from build123d import *

# Parameters (mm, degrees)
SKETCH1_R               = 2.54
BOSS_EXTRUDE1_DEPTH     = 3.175
CUT_EXTRUDE1_DEPTH      = 114.310823319
CUT_EXTRUDE1_DEPTH_BACK = 114.310823319


with BuildPart() as part:
    # Sketch1 → Boss-Extrude1 (new body)
    with BuildSketch(Plane(origin=(0, 0, 0), x_dir=(1, 0, 0), z_dir=(0, 1, 0))):
        with BuildLine():
            Line((108.539117009, 4.335152614), (5.263477484, 12.318590912))
            ThreePointArc((5.263477484, 12.318590912), (3.157372026, 12.484449553), (1.051753091, 12.656374498))
            ThreePointArc((1.051753091, 12.656374498), (-12.7, 0), (1.051753091, -12.656374498))
            ThreePointArc((1.051753091, -12.656374498), (3.157372026, -12.484449553), (5.263477484, -12.318590912))
            Line((5.263477484, -12.318590912), (108.539117009, -4.335152614))
            ThreePointArc((108.539117009, -4.335152614), (112.55208597, 0), (108.539117009, 4.335152614))
        make_face()
        with Locations(Location((108.204, 0, 0), (0, 0, 270))):
            Circle(SKETCH1_R, mode=Mode.SUBTRACT)
        with Locations(Location((96.52, 0, 0), (0, 0, 270))):
            Circle(SKETCH1_R, mode=Mode.SUBTRACT)
        with Locations(Location((84.836, 0, 0), (0, 0, 270))):
            Circle(SKETCH1_R, mode=Mode.SUBTRACT)
    extrude(amount=BOSS_EXTRUDE1_DEPTH)

    # Sketch3 → Cut-Extrude1 (cut, two sides: drawn at the far end of the back side and taken through both)
    with BuildSketch(Plane(origin=(0, 0, 0), x_dir=(1, 0, 0), z_dir=(0, 1, 0)).offset(-CUT_EXTRUDE1_DEPTH_BACK)):
        with BuildLine():
            Line((-4.018100173, 8.636), (4.018100173, 8.636))
            ThreePointArc((4.018100173, 8.636), (0, -9.525), (-4.018100173, 8.636))
        make_face()
    extrude(amount=CUT_EXTRUDE1_DEPTH + CUT_EXTRUDE1_DEPTH_BACK, mode=Mode.SUBTRACT)


solid = part.part
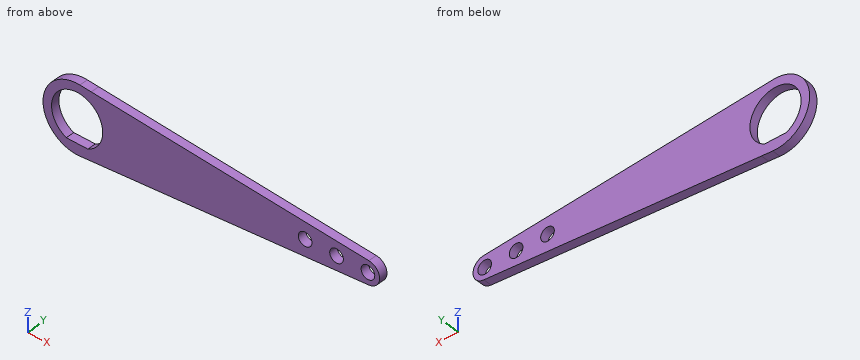
The model under review builds one solid part; all positions refer to its coordinate system, in mm. Give positions to 0.01 mm unless a question says otherwise; leave off trailing zeros. Loops run counter-clockwise (first coordinate to the right, second up) from the corner with the lowest first, then second, coordinate; pieces in that order, holes last. Notation, with made-up numbers: (-33.75, 2.5) -> (3.25, 2.5) arc R15 ccw to (3.25, 25.5) -> close; hole circle Ø9 at (15.5, -20). An arc over 180 degrees is marked (long way). Answer as a JSON object with one key per item and string values. Group by question number.
Q1. Take a section at D-D (z = 6.75). Write out the cut boundary in (x, y) (3 decimals), plus the area to 3 significant figures.
Q2. Wall thickness on line 1 along X through (y, z) = (1.2, 0) (3 decimals); line 2 along X through (y, z) = (2.2, 2); line 3 along Z through (x, y) = (0, 0.9) (3 decimals): over which ranges is each line inside the solid? List them lowest first.
Q3. Insertion check: pin 1 (8 mm diameter, centred on x = 96.52, z = 0, fed in from -Y); pin 2 (1.5 mm diameter, centred on y = 1.5, z = 1.5, fed in from +X); pin 3 (1.6 mm diameter, centred on x = -1.5, y = 2.5, fed in from +Z); pin 4 (1.5 mm diameter, centred on x = 50.5, y = 1.5, fed in from -Z). Each pin has a flat end and moves straight along its axis. Give the tip position at first contact, or say it passes through.
Q4. Take a section at A-A (x = 0). Write out the cut boundary in (y, z) (3 decimals).
Q5. Take a section at B-B (z = 0). Write out the cut boundary in (x, y) (3 decimals).
Q6. Take a section at C-C (y = 2.65). Write out the cut boundary in (x, z) (3 decimals), plus the area to 3 significant figures.
Answer below:
{
 "1": {"outline": "(-10.758, 0) -> (-6.72, 0) -> (-6.72, 3.175) -> (-10.758, 3.175) -> close; (6.72, 0) -> (77.3, 0) -> (77.3, 3.175) -> (6.72, 3.175) -> close", "area": "237 mm2"},
 "2": {"line 1": "x = -12.7 to -9.525, 9.525 to 82.296, 87.376 to 93.98, 99.06 to 105.664, 110.744 to 112.552", "line 2": "x = -12.54 to -9.31, 9.31 to 83.27, 86.4 to 94.95, 98.09 to 106.64, 109.77 to 112.06", "line 3": "z = -12.7 to -8.636, 9.525 to 12.7"},
 "3": {"pin 1": "stops at y = 0", "pin 2": "stops at x = 112.49", "pin 3": "stops at z = 12.68", "pin 4": "stops at z = -8.88"},
 "4": {"outline": "(0, -12.7) -> (3.175, -12.7) -> (3.175, -8.636) -> (0, -8.636) -> close; (0, 9.525) -> (3.175, 9.525) -> (3.175, 12.7) -> (0, 12.7) -> close"},
 "5": {"outline": "(-12.7, 0) -> (-9.525, 0) -> (-9.525, 3.175) -> (-12.7, 3.175) -> close; (9.525, 0) -> (82.296, 0) -> (82.296, 3.175) -> (9.525, 3.175) -> close; (87.376, 0) -> (93.98, 0) -> (93.98, 3.175) -> (87.376, 3.175) -> close; (99.06, 0) -> (105.664, 0) -> (105.664, 3.175) -> (99.06, 3.175) -> close; (110.744, 0) -> (112.552, 0) -> (112.552, 3.175) -> (110.744, 3.175) -> close"},
 "6": {"outline": "(1.052, -12.656) arc R733.38 cw to (5.263, -12.319) -> (108.539, -4.335) arc R4.348 ccw to (108.539, 4.335) -> (5.263, 12.319) arc R733.38 cw to (1.052, 12.656) arc R12.7 ccw (long way) to start; hole (-4.018, -8.636) -> (4.018, -8.636) arc R9.525 ccw (long way) to start; hole circle Ø5.08 at (84.836, 0); hole circle Ø5.08 at (96.52, 0); hole circle Ø5.08 at (108.204, 0)", "area": "1,790 mm2"}
}
